from build123d import *

# Parameters (mm, degrees)
SKETCH1_R               = 154.305
BOSS_EXTRUDE1_DEPTH     = 25.4
SKETCH3_R               = 3.37312
CUT_EXTRUDE1_DEPTH      = 276.403891776
SKETCH5_R               = 25.4
CUT_EXTRUDE2_DEPTH      = 276.403891776
SKETCH6_W               = 159.004
SKETCH6_H               = 159.004
CUT_EXTRUDE3_DEPTH      = 19.05
BOSS_EXTRUDE2_START     = -19.05
SKETCH7_R               = 158.75
SKETCH7_R_2             = 154.305
BOSS_EXTRUDE2_DEPTH     = 44.45
CUT_EXTRUDE4_DEPTH      = 4.9276
CUT_EXTRUDE8_REACH      = 266.23
CUT_EXTRUDE8_END_RADIUS = 25.4
SKETCH11_R              = 2.499995
CUT_EXTRUDE9_DEPTH      = 8.0000094
BOSS_EXTRUDE3_START     = 19.05
SKETCH12_R              = 29.21
SKETCH12_R_2            = 25.4
BOSS_EXTRUDE3_DEPTH     = 19.05
FILLET1_R               = 1.905


with BuildPart() as part:
    # Sketch1 → Boss-Extrude1 (new body)
    with BuildSketch(Plane(origin=(0, 0, 0), x_dir=(1, 0, 0), z_dir=(0, 1, 0))):
        with Locations(Location((0, 0, 0), (0, 0, 270))):
            Circle(SKETCH1_R)
    extrude(amount=BOSS_EXTRUDE1_DEPTH)

    # Sketch3 → Cut-Extrude1 (cut, through all)
    with BuildSketch(Plane(origin=(3.2638069, 0, 70.137007426), x_dir=(-1, 0, 0), z_dir=(0, -1, 0))):
        with Locations(Location((-67.3799431, 140.780757426, 0), (0, 0, 90))):
            Circle(SKETCH3_R)
        with Locations(Location((73.9075569, 140.780757426, 0), (0, 0, 90))):
            Circle(SKETCH3_R)
        with Locations(Location((73.9075569, -0.506742574, 0), (0, 0, 90))):
            Circle(SKETCH3_R)
        with Locations(Location((-67.3799431, -0.506742574, 0), (0, 0, 90))):
            Circle(SKETCH3_R)
    extrude(amount=-CUT_EXTRUDE1_DEPTH, mode=Mode.SUBTRACT)

    # Sketch5 → Cut-Extrude2 (cut, through all)
    with BuildSketch(Plane(origin=(3.2638069, 0, 70.137007426), x_dir=(-1, 0, 0), z_dir=(0, -1, 0))):
        with Locations(Location((3.2638069, 70.137007426, 0), (0, 0, 90))):
            Circle(SKETCH5_R)
    extrude(amount=-CUT_EXTRUDE2_DEPTH, mode=Mode.SUBTRACT)

    # Sketch6 → Cut-Extrude3 (cut)
    with BuildSketch(Plane.XZ):
        Rectangle(SKETCH6_W, SKETCH6_H)
    extrude(amount=-CUT_EXTRUDE3_DEPTH, mode=Mode.SUBTRACT)

    # Sketch7 → Boss-Extrude2 (add)
    with BuildSketch(Plane(origin=(0, 0, 0), x_dir=(1, 0, 0), z_dir=(0, 1, 0)).offset(BOSS_EXTRUDE2_START)):
        with Locations(Location((0, 0, 0), (0, 0, 270))):
            Circle(SKETCH7_R)
        with Locations(Location((0, 0, 0), (0, 0, 270))):
            Circle(SKETCH7_R_2, mode=Mode.SUBTRACT)
    extrude(amount=BOSS_EXTRUDE2_DEPTH)

    # Sketch8 → Cut-Extrude4 (cut)
    with BuildSketch(Plane(origin=(0, 25.4, 0), x_dir=(1, 0, 0), z_dir=(0, 1, 0))):
        with BuildLine():
            Line((-10.642138235, -102.903613136), (-10.642138235, -50.942074053))
            ThreePointArc((-10.642138235, -50.942074053), (0, -40.299935817), (10.642138235, -50.942074053))
            Line((10.642138235, -50.942074053), (10.642138235, -102.903613136))
            ThreePointArc((10.642138235, -102.903613136), (0, -113.545751371), (-10.642138235, -102.903613136))
        make_face()
    extrude(amount=-CUT_EXTRUDE4_DEPTH, mode=Mode.SUBTRACT)

    # Cut-Extrude8: up to this cylinder (the profile starts outside it)
    cut_extrude8_end = Plane(origin=(0, 22.143059, 0), z_dir=(0, -1, 0)) * Cylinder(CUT_EXTRUDE8_END_RADIUS, 584.26, mode=Mode.PRIVATE)
    # Sketch10 → Cut-Extrude8 (cut, up to the surface)
    with BuildSketch(Plane(origin=(0, 0, 50.942074053), x_dir=(-1, 0, 0), z_dir=(0, 0, -1)), mode=Mode.PRIVATE) as cut_extrude8_sk1:
        with BuildLine():
            Line((3.978866006, 20.464038844), (-3.978866006, 20.464038844))
            ThreePointArc((-3.978866006, 20.464038844), (0, 24.421873778), (3.978866006, 20.464038844))
        make_face()
    cut_extrude8_tool1 = extrude(cut_extrude8_sk1.sketch, amount=CUT_EXTRUDE8_REACH, mode=Mode.PRIVATE) - cut_extrude8_end
    add(cut_extrude8_tool1.solids().sort_by_distance((0, 22.143059, 50.942074))[0], mode=Mode.SUBTRACT)

    # Sketch11 → Cut-Extrude9 (cut)
    with BuildSketch(Plane(origin=(0, 25.4, 0), x_dir=(1, 0, 0), z_dir=(0, 1, 0))):
        with Locations(Location((-38.1, -64.976536144, 0), (0, 0, 270))):
            Circle(SKETCH11_R)
        with Locations(Location((38.1, -64.976536144, 0), (0, 0, 270))):
            Circle(SKETCH11_R)
        with Locations(Location((38.1, -112.910719468, 0), (0, 0, 270))):
            Circle(SKETCH11_R)
        with Locations(Location((-38.1, -112.910719468, 0), (0, 0, 270))):
            Circle(SKETCH11_R)
    extrude(amount=-CUT_EXTRUDE9_DEPTH, mode=Mode.SUBTRACT)

    # Sketch12 → Boss-Extrude3 (add)
    with BuildSketch(Plane.XZ.offset(-19.05).offset(BOSS_EXTRUDE3_START)):
        with Locations(Location((0, 0, 0), (0, 0, 90))):
            Circle(SKETCH12_R)
        with Locations(Location((0, 0, 0), (0, 0, 270))):
            Circle(SKETCH12_R_2, mode=Mode.SUBTRACT)
    extrude(amount=-BOSS_EXTRUDE3_DEPTH)

    # Fillet1
    # the kernel refuses this fillet: 1.905 mm, written as the material it adds along each edge
    with BuildSketch(Plane(origin=(0, 19.05, 0), x_dir=(0, 0, 1), z_dir=(1, 0, 0))) as fillet1_piece_1:
        with BuildLine():
            CenterArc((29.21 + FILLET1_R, FILLET1_R), FILLET1_R, 180, 90)
            Line((29.21, FILLET1_R), (29.21, 0))
            Line((29.21, 0), (29.21 + FILLET1_R, 0))
        make_face()
    revolve(axis=Axis((0, 19.05, 0), (0, -1, 0)))
    # the kernel refuses this fillet: 1.905 mm, written as the material it takes off along each edge
    with BuildSketch(Plane(origin=(0, 0, 0), x_dir=(0, 0, -1), z_dir=(-1, 0, 0))) as fillet1_2_piece_1:
        with BuildLine():
            CenterArc((25.4 + FILLET1_R, -FILLET1_R), FILLET1_R, 90, 90)
            Line((25.4 + FILLET1_R, 0), (25.4, 0))
            Line((25.4, 0), (25.4, -FILLET1_R))
        make_face()
    revolve(axis=Axis((0, 0, 0), (0, -1, 0)), mode=Mode.SUBTRACT)
    with BuildSketch(Plane(origin=(-10.642138235, 25.4, 102.903613136), x_dir=(-1, 0, 0), z_dir=(0, 0, -1)), Plane(origin=(10.642138235, 25.4, 50.942074053), x_dir=(1, 0, 0), z_dir=(0, 0, 1))) as fillet1_2_piece_2:
        with BuildLine():
            CenterArc((FILLET1_R, -FILLET1_R), FILLET1_R, 90, 90)
            Line((0, -FILLET1_R), (0, 0))
            Line((0, 0), (FILLET1_R, 0))
        make_face()
    extrude(amount=51.961539084, mode=Mode.SUBTRACT)
    with BuildSketch(Plane(origin=(0, 25.4, 102.903613136), x_dir=(1, 0, 0), z_dir=(0, 0, -1))) as fillet1_2_piece_3:
        with BuildLine():
            CenterArc((10.642138235 + FILLET1_R, FILLET1_R), FILLET1_R, 180, 90)
            Line((10.642138235, FILLET1_R), (10.642138235, 0))
            Line((10.642138235, 0), (10.642138235 + FILLET1_R, 0))
        make_face()
    revolve(axis=Axis((0, 25.4, 102.903613136), (0, -1, 0)), revolution_arc=180, mode=Mode.SUBTRACT)
    with BuildSketch(Plane(origin=(0, 25.4, 50.942074053), x_dir=(-1, 0, 0), z_dir=(0, 0, 1))) as fillet1_2_piece_4:
        with BuildLine():
            CenterArc((10.642138235 + FILLET1_R, FILLET1_R), FILLET1_R, 180, 90)
            Line((10.642138235, FILLET1_R), (10.642138235, 0))
            Line((10.642138235, 0), (10.642138235 + FILLET1_R, 0))
        make_face()
    revolve(axis=Axis((0, 25.4, 50.942074053), (0, -1, 0)), revolution_arc=180, mode=Mode.SUBTRACT)
    with BuildSketch(Plane(origin=(0, 20.464038844, 0), x_dir=(0.33800763161773084, 0, 0.9411433689763598), z_dir=(0.9411433689763598, 0, -0.33800763161773084))) as fillet1_2_piece_5_section:
        with BuildLine():
            CenterArc((25.4 + FILLET1_R, FILLET1_R), FILLET1_R, 180, 90)
            Line((25.4 + FILLET1_R, 0), (25.4, 0))
            Line((25.4, 0), (25.4, FILLET1_R))
        make_face()
    fillet1_2_piece_5 = revolve(axis=Axis((0, 20.464038844, 0), (0, -1, 0)), revolution_arc=39.511069251, mode=Mode.PRIVATE)
    fillet1_2_piece_5 = fillet1_2_piece_5 & Plane(origin=(0, 20.442951895, 25.734088131), x_dir=(0.9999859566813862, 0.0052996641415057515, 0), z_dir=(0, 0, 1)) * Cylinder(3.978921884, 110, mode=Mode.PRIVATE)
    add(fillet1_2_piece_5, mode=Mode.SUBTRACT)


solid = part.part
Input: part model. Units: mm. Frame: model coordinates. A direction names the side the tool comes from. Give positions to 0.01 mm unless a question says otherwise; leave off trailing zeros. Order: outer loops, then holes, each group sorted by start corner. A loop starts at its lowest first (then second) coordinate and runs counter-clockwise, first axis right, second up. Notation, with made-up numbers: (57, 80.25) - (67, 80.25) arc R33 ccw to (67, 116.25) - close; hole circle Ø5 at (3, -4). An arc over 180 degrees is marked (long way). Answer as a JSON object with one key per item and string values. Group by question number.
Q1. Cut plane A-A, the plane y = 7.5. Output: boundary loops of the cut face in (x, z).
Q2. Set-up query: faces 4 (the face through (7.629, 13.488, -24.227)), 5 (the face through (0, 20.464, 39)), 6 (the face through (-79.502, 9, -1)), 7 (the face through (8.318, 22.005, 44.304)). Return all of +Z, -Z, +X, -X, +Y, -Y with unobstructed straight access to the full face (end or side cutting, diameter ignored); none if empty.
Q3. Line query: probe 1 along Z at (x, y) = (1.5, 5.5); probe 2 along X at (y, z) = (-9, 4); probe 3 along X at (y, z) = (-6, 0) (3 decimals). Output: solid intervals per line, ascending.
Q4. Cut plane B-B, the plane z = 0. Output: boundary loops of the cut face in (x, y) (3 decimals).
Q5. Cut plane D-D, the plane z = -54. Output: boundary loops of the cut face in (x, y).
Q6. First-contact query: pin 1 Ø9.5 at (y, z) = (5.5, -11) entering from +X; pin 2 Ø2 at (y, z) = (-14, 70.5) entering from -X; pin 3 Ø1 at (x, y) = (-126, 20.5) entering from -Z. Flat tips, straight axial feed; report the tip coordinate or a pass-through.
Q7. Cut plane C-C, the plane x = 56. Output: boundary loops of the cut face in (y, z), then the cut area to 3 significant figures.
Q8. Mould query, pull axis Z, two halves, no side actions, for faces 1 (the face through (47.68, 2.86, 151.42)), 2 (the face through (-24.63, 8.45, 15.7)), 3 (the face through (-33, 25.4, -2)). Classes: pulls with the +Z half, pulls with the -Z half, needs draft (parallel to the pull), parting line crosses it, or undercut.
Results:
{
 "1": {"outline": "circle Ø317.5 at (0, 0); circle Ø58.42 at (0, 0); hole (-79.5, -79.5) - (79.5, -79.5) - (79.5, 79.5) - (-79.5, 79.5) - close; hole circle Ø50.8 at (0, 0)"},
 "2": {"face 4": "+Y, -Y", "face 5": "none", "face 6": "-Y", "face 7": "+Y"},
 "3": {"probe 1": "-158.74 to -79.5, -29.17 to -25.36, 25.36 to 29.17, 79.5 to 158.74", "probe 2": "-158.7 to -154.25, 154.25 to 158.7", "probe 3": "-158.75 to -154.305, 154.305 to 158.75"},
 "4": {"outline": "(-158.75, -19.05) - (-154.305, -19.05) - (-154.305, 0) - (-79.502, 0) - (-79.502, 19.05) - (-31.115, 19.05) arc R1.905 cw to (-29.21, 17.145) - (-29.21, 0) - (-27.305, 0) arc R1.905 ccw to (-25.4, 1.905) - (-25.4, 25.4) - (-158.75, 25.4) - close; (25.4, 1.905) arc R1.905 ccw to (27.305, 0) - (29.21, 0) - (29.21, 17.145) arc R1.905 cw to (31.115, 19.05) - (79.502, 19.05) - (79.502, 0) - (154.305, 0) - (154.305, -19.05) - (158.75, -19.05) - (158.75, 25.4) - (25.4, 25.4) - close"},
 "5": {"outline": "(-149.28, -19.05) - (-144.55, -19.05) - (-144.55, 0) - (-79.5, 0) - (-79.5, 19.05) - (79.5, 19.05) - (79.5, 0) - (144.55, 0) - (144.55, -19.05) - (149.28, -19.05) - (149.28, 25.4) - (-149.28, 25.4) - close"},
 "6": {"pin 1": "x = 158.63", "pin 2": "x = -142.73", "pin 3": "z = -97.22"},
 "7": {"outline": "(-19.05, -148.54) - (25.4, -148.54) - (25.4, 148.54) - (-19.05, 148.54) - (-19.05, 143.78) - (0, 143.78) - (0, 79.5) - (19.05, 79.5) - (19.05, -79.5) - (0, -79.5) - (0, -143.78) - (-19.05, -143.78) - close", "area": "4,700 mm^2"},
 "8": {"face 1": "parting line crosses it", "face 2": "undercut", "face 3": "needs draft"}
}
